```python
from build123d import *

# Parameters (mm, degrees)
BOSS_EXTRUDE1_DEPTH = 20


with BuildPart() as part:
    # Sketch2 → Boss-Extrude1 (new body)
    with BuildSketch(Plane(origin=(0, 0, 0), x_dir=(1, 0, 0), z_dir=(0, 1, 0))):
        with BuildLine():
            Line((-10, 0), (-10, -10))
            ThreePointArc((-10, -10), (0, -20), (10, -10))
            Line((10, -10), (10, 0))
            Line((10, 0), (30, 0))
            Line((30, 0), (30, -30))
            Line((30, -30), (-30, -30))
            Line((-30, -30), (-30, 0))
            Line((-30, 0), (-10, 0))
        make_face()
    extrude(amount=BOSS_EXTRUDE1_DEPTH)


solid = part.part
```
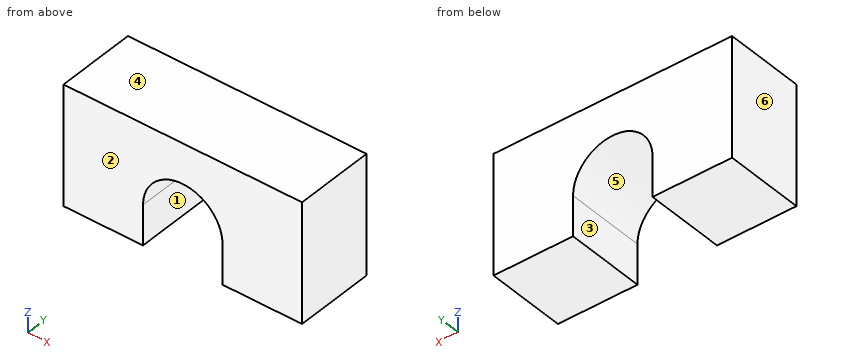
Input: part model. Units: mm. Frame: model coordinates. Face numbers are marked on the shaded views. A direction names the side the tool comes from. Round coordinates to 2 decimals unless told otherwise and drop trailing zeros. Order: outer loops, then holes, each group sorted by start corner. A loop starts at its lowest first (then second) coordinate and runs counter-clockwise, first axis right, second up. Notation, with made-up numbers: (76.5, 10.25) - (120.5, 10.25) arc R21 cw to (120.5, 18.25) - close; hole circle Ø10 at (51, 60.25). An arc over 180 degrees is marked (long way). One line per question, with ' | ' between items. Start each with the question number.
1) Set-up query: the marked faces 1 and 2. Return all of +Z, -Z, +X, -X, +Y, -Y with unobstructed straight access to the full face (end or side cutting, diameter ignored); none if empty.
2) Cut plane B-B, the plane y = 7.5. Return the cut outline in (x, z), then the cut area to 3 significant figures.
3) Pull-direction query (X, two-part tool) for the marked faces 3, 4, 5 and 6; classes: +X half, -X half, draft (parallel to the pull), parting line (faces both ways), or undercut.
4) Cut plane C-C, the plane x = 0. Return the cut outline in (y, z).
5) Ray query, probe 1 along X at (y, z) = (5, 2.75); probe 2 along X at (y, z) = (15, 14.5); probe 3 along Z at (x, y) = (2.5, 11). Return the intervals inside material, ascending.
6) Cut plane A-A, the plane z = 10.75. Return the cut outline in (x, y), then the cut area to 3 significant figures.
7) Contact query for flat-ended pins moving along their axis: P1, Ø5, axis at x = -3, y = 7.5, coming from the -Z side; P2, Ø8, axis at x = -7.5, z = 9, coming from the -Y side. Output: stop coordinate, or through.
Worked out:
1) face 1: -Z, +Y, -Y | face 2: +Z, -Z, +X, -X, -Y
2) outline: (-30, 0) - (-10, 0) - (-10, 10) arc R10 cw to (10, 10) - (10, 0) - (30, 0) - (30, 30) - (-30, 30) - close | area: 1,440 mm^2
3) face 3: undercut | face 4: draft | face 5: undercut | face 6: -X half
4) outline: (0, 20) - (20, 20) - (20, 30) - (0, 30) - close
5) probe 1: x = -30 to -10, 10 to 30 | probe 2: x = -30 to -8.93, 8.93 to 30 | probe 3: z = 19.68 to 30
6) outline: (-30, 0) - (-9.97, 0) - (-9.97, 20) - (-30, 20) - close; (9.97, 0) - (30, 0) - (30, 20) - (9.97, 20) - close | area: 801 mm^2
7) P1: stops at z = 18.35 | P2: stops at y = 0
